Source: CAD feature listing. Evaluate the final solid. Frame: model axes, mm. Face numbers are marked on the shaded views. A direction names the side the tool comes from. Round coordinates to 2 decimals unless told otherwise and drop trailing zeros. Write each loop counter-clockwise with the first axis right and the second up, starting at its lowest first coordinate (ties: lowest second). Pieces come first, ordered by that corner, then holes. Notation, with made-up numbers: (42, 24.5) -> (101, 24.5) arc R25 cw to (101, 53.5) -> close; hole circle Ø2 at (54.25, 15). An arc over 180 degrees is marked (long way). Return JSON: item names as keys, results as strings. Group by question number.
from build123d import *

# Parameters (mm, degrees)
EXTRUDE_1_DEPTH     = 45
CUT_EXTRUDE_1_DEPTH = 33
SKETCH_3_R          = 11.25
CUT_EXTRUDE_2_DEPTH = 13
SKETCH_4_R          = 1.65
CUT_EXTRUDE_3_DEPTH = 13
SKETCH_5_R          = 3
CUT_EXTRUDE_4_DEPTH = 11
SKETCH_6_R          = 5
CUT_EXTRUDE_5_DEPTH = 5
SKETCH_7_R          = 15
CUT_EXTRUDE_6_DEPTH = 8


with BuildPart() as part:
    # Эскиз1 → Бобышка-Вытянуть1 (new body)
    with BuildSketch(Plane(origin=(0, 0, 0), x_dir=(1, 0, 0), z_dir=(0, 1, 0))):
        Polygon((-21.15, 21.15), (21.15, 21.15), (41.15, 21.15), (41.15, 11.15), (25, 11.15), (25, -25), (-25, -25), (-25, 11.15), (-41.15, 11.15), (-41.15, 21.15), align=None)
    extrude(amount=EXTRUDE_1_DEPTH)

    # Эскиз2 → Вырез-Вытянуть1 (cut)
    with BuildSketch(Plane.XZ):
        Polygon((-21.5, 16.5), (-16.5, 21.5), (16.5, 21.5), (21.5, 16.5), (21.5, -21.5), (-21.5, -21.5), align=None)
    extrude(amount=-CUT_EXTRUDE_1_DEPTH, mode=Mode.SUBTRACT)

    # Эскиз3 → Вырез-Вытянуть2 (cut, through all)
    with BuildSketch(Plane.XZ.offset(-33)):
        Circle(SKETCH_3_R)
    extrude(amount=-CUT_EXTRUDE_2_DEPTH, mode=Mode.SUBTRACT)

    # Эскиз4 → Вырез-Вытянуть3 (cut, through all)
    with BuildSketch(Plane.XZ.offset(-33)):
        with Locations((-15.5, 15.5)):
            Circle(SKETCH_4_R)
        with Locations((15.5, 15.5)):
            Circle(SKETCH_4_R)
        with Locations((-15.5, -15.5)):
            Circle(SKETCH_4_R)
        with Locations((15.5, -15.5)):
            Circle(SKETCH_4_R)
    extrude(amount=-CUT_EXTRUDE_3_DEPTH, mode=Mode.SUBTRACT)

    # Эскиз5 → Вырез-Вытянуть4 (cut, through all)
    with BuildSketch(Plane.XY.offset(-11.15)):
        with Locations((-33.075, 22.5)):
            Circle(SKETCH_5_R)
        with Locations((33.075, 22.5)):
            Circle(SKETCH_5_R)
    extrude(amount=-CUT_EXTRUDE_4_DEPTH, mode=Mode.SUBTRACT)

    # Эскиз6 → Вырез-Вытянуть5 (cut)
    with BuildSketch(Plane.XY.offset(-11.15)):
        with Locations((-33.075, 22.5)):
            Circle(SKETCH_6_R)
        with Locations((33.075, 22.5)):
            Circle(SKETCH_6_R)
    extrude(amount=-CUT_EXTRUDE_5_DEPTH, mode=Mode.SUBTRACT)

    # Эскиз7 → Вырез-Вытянуть6 (cut)
    with BuildSketch(Plane(origin=(0, 45, 0), x_dir=(1, 0, 0), z_dir=(0, 1, 0))):
        Circle(SKETCH_7_R)
    extrude(amount=-CUT_EXTRUDE_6_DEPTH, mode=Mode.SUBTRACT)


solid = part.part
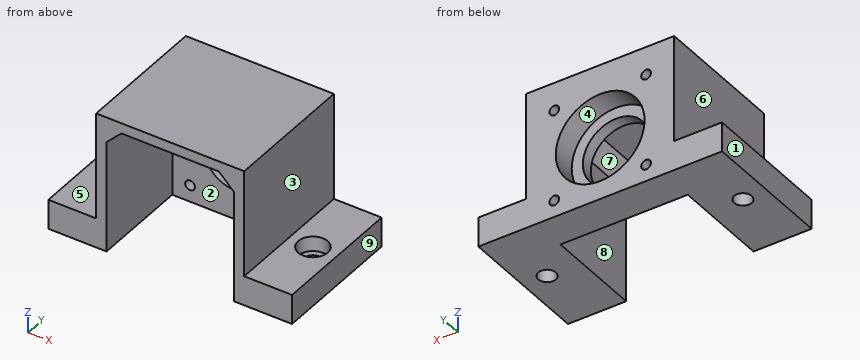
Item 1: Pull-direction query (X, two-part tool) for the marked faces 6, 7, 8 and 9; classes: +X half, -X half, draft (parallel to the pull), parting line (faces both ways), or undercut.
Item 2: First-contact query: pin 1 Ø18 at (y, z) = (12.5, 5) entering from -X; pin 2 Ø12 at (x, z) = (0.5, 4.5) entering from +Y; pin 3 Ø11 at (x, y) = (-35, 23) entering from +Z; pin 4 Ø1.5 at (y, z) = (7.5, -1) entering from +X. Flat tips, straight axial feed; report the tip coordinate or a pass-through.
Item 3: Material intervals for probe 1 along Z at (x, y) = (15.5, 41); probe 2 along X at (y, z) = (14.5, 3.5); probe 3 along X at (y, z) = (36.5, 16.5), sorted ascending.
Item 4: Cut plane C-C on y = 22.5. Give the number of separate pieces and of enclosed holes in the cut face, and give its area (3 significant figures).
Item 5: Set-up query: the marked faces 1, 2, 3, 4 and 5. Return all of +Z, -Z, +X, -X, +Y, -Y with unobstructed straight access to the full face (end or side cutting, diameter ignored); none if empty.
Item 6: Cut plane A-A on x = 0. Output: boundary loops of the cut face in (y, z), and give its area (3 significant figures).
Item 7: Cut plane B-B on z = -9. Output: boundary loops of the cut face in (x, y).
Item 8: Cut plane D-D on y = 30.5. Output: boundary loops of the cut face in (x, z).
Here are the results:
{
 "1": {"face 6": "-X half", "face 7": "undercut", "face 8": "undercut", "face 9": "+X half"},
 "2": {"pin 1": "stops at x = -25", "pin 2": "passes through", "pin 3": "stops at z = -11.15", "pin 4": "stops at x = 25"},
 "3": {"probe 1": "z = -21.15 to -17.15, -13.85 to 13.85, 17.15 to 25", "probe 2": "x = -25 to -21.5, 21.5 to 25", "probe 3": "x = -25 to -16.81, -14.19 to 14.19, 16.81 to 25"},
 "4": {"separate pieces": "3", "enclosed holes": "0", "area": "662 mm^2"},
 "5": {"face 1": "+Z, -Z, -X, +Y, -Y", "face 2": "-Z, -Y", "face 3": "+Z, +X, +Y, -Y", "face 4": "+Y", "face 5": "+Z, -X, +Y, -Y"},
 "6": {"outline": "(0, 21.5) -> (33, 21.5) -> (33, 11.25) -> (37, 11.25) -> (37, 15) -> (45, 15) -> (45, 25) -> (0, 25) -> close; (33, -21.15) -> (45, -21.15) -> (45, -15) -> (37, -15) -> (37, -11.25) -> (33, -11.25) -> close", "area": "339 mm^2"},
 "7": {"outline": "(-25, 0) -> (-21.5, 0) -> (-21.5, 33) -> (-6.75, 33) -> (-6.75, 37) -> (-12, 37) -> (-12, 45) -> (-25, 45) -> close; (6.75, 33) -> (21.5, 33) -> (21.5, 0) -> (25, 0) -> (25, 45) -> (12, 45) -> (12, 37) -> (6.75, 37) -> close"},
 "8": {"outline": "(-41.15, -21.15) -> (-21.5, -21.15) -> (-21.5, 16.5) -> (-16.5, 21.5) -> (16.5, 21.5) -> (21.5, 16.5) -> (21.5, -21.15) -> (41.15, -21.15) -> (41.15, -11.15) -> (25, -11.15) -> (25, 25) -> (-25, 25) -> (-25, -11.15) -> (-41.15, -11.15) -> close"}
}
